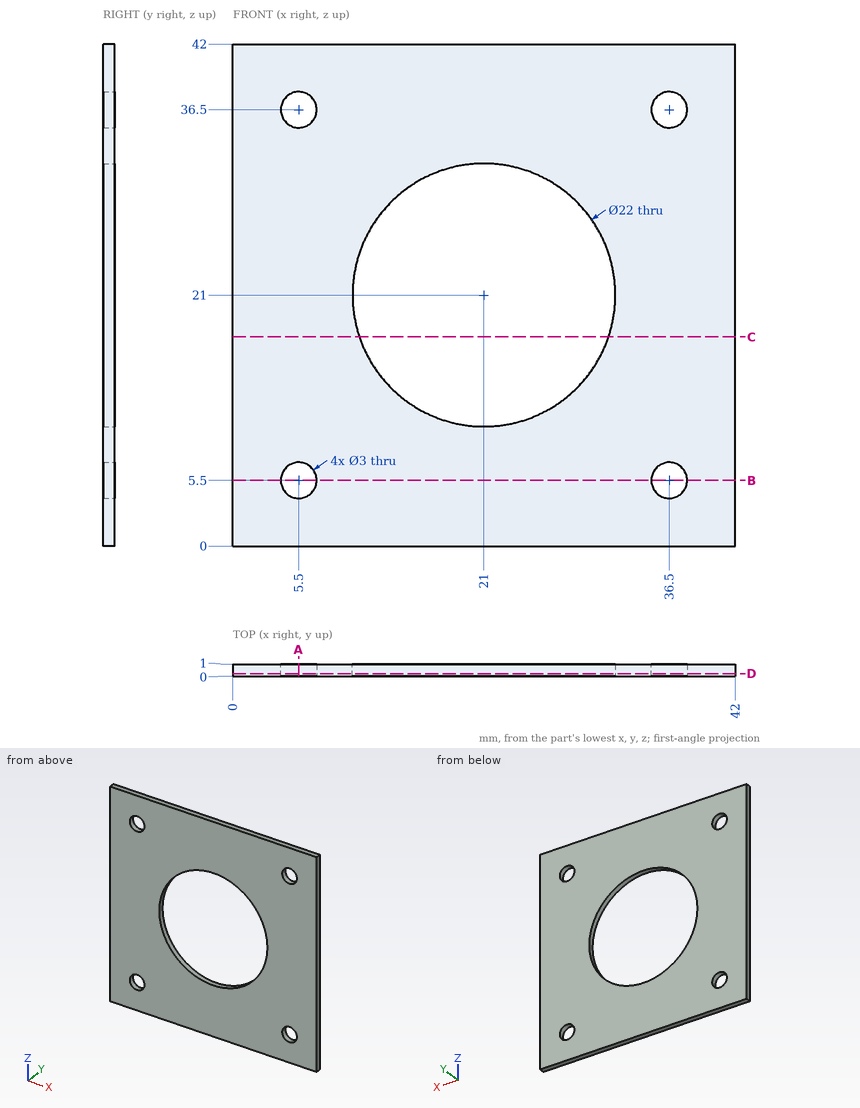
The drawing under review shows one solid part. Ordinate dimensions are in mm from its lowest x, y, z. Round coordinates to 2 decimals unless told otherwise and drop trailing zeros. Loops run counter-clockwise (first coordinate to the right, second up) from the corner with the lowest first, then second, coordinate; pieces in that order, holes last. Notation, with made-up numbers: (-3.5, 42.5) - (13.5, 42.5) arc R24 cw to (13.5, 61.5) - close; hole circle Ø7 at (59, 61.25). An arc over 180 degrees is marked (long way). Put each result on its own line as item: value. Start each with the question number.
1. Insertion check: P1, Ø4, axis at x = 28.5, z = 37.5, coming from the -Y side. The pin has a flat end and moves straight along its axis. Give the tip position at first contact, or say it passes through.
2. For probe 1 along Z at (x, y) = (36.5, 0.5); probe 2 along Z at (x, y) = (21, 0.2); probe 3 along Z at (x, y) = (5, 0.35), list the stretches that pass through material, from the lowest coordinate up. Write a range as [from, to].
3. Consider section D-D on y = 0.2. State the section outline as (x, z) points.
4. Consider section C-C on z = 17.5. State the section outline as (x, y) points.
5. Consider section B-B on z = 5.5. State the section outline as (x, y) points.
6. Consider section A-A on x = 5.5. State the section outline as (y, z) points, plus the area to 3 significant figures.
Result sheet:
1. P1: y = 0
2. probe 1: [0, 4], [7, 35], [38, 42]
2. probe 2: [0, 10], [32, 42]
2. probe 3: [0, 4.09], [6.91, 35.09], [37.91, 42]
3. outline: (0, 0) - (42, 0) - (42, 42) - (0, 42) - close; hole circle Ø3 at (5.5, 5.5); hole circle Ø3 at (5.5, 36.5); hole circle Ø22 at (21, 21); hole circle Ø3 at (36.5, 5.5); hole circle Ø3 at (36.5, 36.5)
4. outline: (0, 0) - (10.57, 0) - (10.57, 1) - (0, 1) - close; (31.43, 0) - (42, 0) - (42, 1) - (31.43, 1) - close
5. outline: (0, 0) - (4, 0) - (4, 1) - (0, 1) - close; (7, 0) - (35, 0) - (35, 1) - (7, 1) - close; (38, 0) - (42, 0) - (42, 1) - (38, 1) - close
6. outline: (0, 0) - (1, 0) - (1, 4) - (0, 4) - close; (0, 7) - (1, 7) - (1, 35) - (0, 35) - close; (0, 38) - (1, 38) - (1, 42) - (0, 42) - close
6. area: 36.0 mm^2
